Could you check a few things on this model? Use its own coordinates, in mm. A direction names the side the tool comes from. Round coordinates to 2 decimals unless told otherwise and drop trailing zeros. Loops run counter-clockwise (first coordinate to the right, second up) from the corner with the lowest first, then second, coordinate; pieces in that order, holes last. Notation, with made-up numbers: (65.5, 62) -> (72.5, 62) arc R26 ccw to (72.5, 94) -> close; hole circle Ø8 at (57.25, 52). An arc over 180 degrees is marked (long way). Put each result on its own line as item: value. Start each with the question number.
1. Imagine slicing it at A-A, the plane z = -45. Please give me the cut outline in (x, y).
2. If we mould it in two halves opening along Z, with no side actions, what happens to faces 1 (the flat face through (4, 30, -54.61)), 2 (the flat face through (4, 30, -36.449)), 3 (the flat face through (10, -9.5, -76)), 4 (the flat face through (4, 30, -13.716))? For each: pulls with the +Z half, pulls with the -Z half, needs draft (parallel to the pull), parting line crosses it, or undercut.
3. Which directions (+Z, -Z, +X, -X, +Y, -Y) give clear straight access to the entire face, cutting with the end or side of a thin tool? Please do faces 5 (the flat face through (1.854, 30, -45)), 6 (the flat face through (60.96, -5, -76)), 7 (the flat face through (4, 30, -59.436)), 8 (the flat face through (68.326, 30, -66)).
4. I'm going to push flat-ended pins straight in: P1, Ø2.5, axis at x = 71.5, y = 31, coming from the +Z side; P2, Ø23, axis at x = 45, z = -57.5, coming from the -Y side; P3, Ø6.5, axis at y = 29, z = -43, coming from the -X side. Where does each tip first touch, or does it pass through?
5. Imagine slicing it at B-B, the plane x = 37. Please give me the cut outline in (y, z), and give its area (3 significant figures).
6. Imagine slicing it at C-C, the plane z = -22. Please give me the cut outline in (x, y).
7. Imagine slicing it at D-D, the plane z = -56. Please give me the cut outline in (x, y).
8. I need wall thicknesses on line 1 (Y direction, x = 27, z = -67.5); line 2 (Z direction, x = 4, y = -1); line 3 (Y direction, x = 71, z = -64). Which ranges of each line are inside material? Lowest first, please. Write a range as [from, to].
```python
from build123d import *

# Parameters (mm, degrees)
SKETCH1_W           = 77.216
SKETCH1_H           = 79.756
BASE_DEPTH          = 25.654
SKETCH2_W           = 5.0038
SKETCH2_H           = 18.161
TOP_HEADERS_DEPTH   = 8.382
SKETCH3_W           = 7.112
SKETCH3_H           = 7.112
SKETCH3_W_2         = 6.5278
BOSS_EXTRUDE3_DEPTH = 9.4996


with BuildPart() as part:
    # Sketch1 → Base (new body)
    with BuildSketch(Plane(origin=(0, 0, 0), x_dir=(1, 0, 0), z_dir=(0, 1, 0))):
        with Locations((38.608, 39.878)):
            Rectangle(SKETCH1_W, SKETCH1_H)
    extrude(amount=BASE_DEPTH)

    # Sketch2 → Top Headers (add)
    with BuildSketch(Plane(origin=(0, 25.654, 0), x_dir=(1, 0, 0), z_dir=(0, 1, 0))):
        with Locations((4.3561, 68.5165)):
            Rectangle(SKETCH2_W, SKETCH2_H)
        with Locations((4.3561, 45.5295)):
            Rectangle(SKETCH2_W, SKETCH2_H)
        with Locations((4.3561, 22.7965)):
            Rectangle(SKETCH2_W, SKETCH2_H)
        with Locations((70.8279, 66.2305)):
            Rectangle(SKETCH2_W, SKETCH2_H)
        with Locations((70.8279, 43.2943)):
            Rectangle(SKETCH2_W, SKETCH2_H)
    extrude(amount=TOP_HEADERS_DEPTH)

    # Sketch3 → Boss-Extrude3 (add)
    with BuildSketch(Plane.XZ):
        with Locations((64.516, -76.2)):
            Rectangle(SKETCH3_W, SKETCH3_H)
        with Locations((9.652, -76.2)):
            Rectangle(SKETCH3_W, SKETCH3_H)
        with Locations((3.8481, -3.556)):
            Rectangle(SKETCH3_W_2, SKETCH3_H)
        with Locations((70.8914, -3.556)):
            Rectangle(SKETCH3_W, SKETCH3_H)
    extrude(amount=BOSS_EXTRUDE3_DEPTH)


solid = part.part
```
Entries:
1. outline: (0, 0) -> (77.22, 0) -> (77.22, 25.65) -> (73.33, 25.65) -> (73.33, 34.04) -> (68.33, 34.04) -> (68.33, 25.65) -> (6.86, 25.65) -> (6.86, 34.04) -> (1.85, 34.04) -> (1.85, 25.65) -> (0, 25.65) -> close
2. face 1: undercut
2. face 2: undercut
2. face 3: needs draft
2. face 4: pulls with the +Z half
3. face 5: +Z, -Z, -X, +Y
3. face 6: +Z, -Z, -Y
3. face 7: -X, +Y
3. face 8: +Z, -Z, +Y
4. P1: z = -34.21
4. P2: y = 0
4. P3: x = 1.85
5. outline: (0, -79.76) -> (25.65, -79.76) -> (25.65, 0) -> (0, 0) -> close
5. area: 2,050 mm^2
6. outline: (0, 0) -> (77.22, 0) -> (77.22, 25.65) -> (6.86, 25.65) -> (6.86, 34.04) -> (1.85, 34.04) -> (1.85, 25.65) -> (0, 25.65) -> close
7. outline: (0, 0) -> (77.22, 0) -> (77.22, 25.65) -> (0, 25.65) -> close
8. line 1: [0, 25.65]
8. line 2: [-7.11, 0]
8. line 3: [0, 34.04]
